Print and shaded views of the part. All mm, measured from the part's lowest x, y and z. Round coordinates to 2 decimals unless told otherwise and drop trailing zeros. Write each loop counter-clockwise with the first axis right and the second up, starting at its lowest first coordinate (ties: lowest second). Pieces come first, ordered by that corner, then holes. Notation, with made-up numbers: (-30, 56) -> (-6, 56) arc R17 cw to (-6, 79) -> close; hole circle Ø3 at (43, 85.25). An arc over 180 degrees is marked (long way). Return JSON: item names as keys, results as strings. Group by question number.
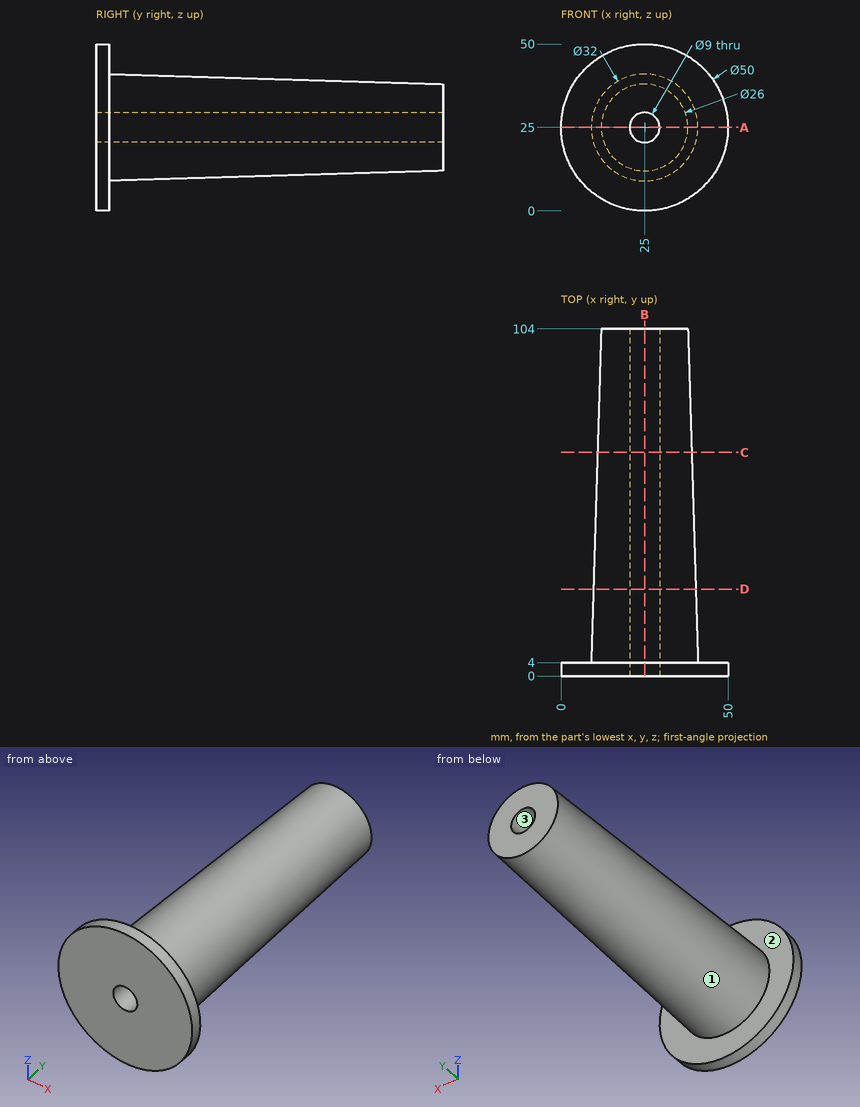
Item 1: Wall check: L1, parallel to Y at x = 39, z = 34; L2, parallel to Z at x = 25, y = 44; L3, parallel to X at y = 33, z = 25. Give the ranges that are in metal, low to high.
Item 2: Cut at C-C (y = 67). Write the cut outline in (x, z).
Item 3: Cut at A-A (z = 25). Write the cut outline in (x, y).
Item 4: Two-plate mould, pull along Z, no slides. Class the marked faces 1, 2 and 3: released by +Z, released by -Z, zero draft, split by the parting line, or undercut.
Item 5: Cut at D-D (y = 26). Write the cut outline in (x, z), then the cut area to 3 significant figures.
Item 6: Flat gauge pins, fed straight in: P1, Ø12, axis at y = 87.5, z = 23.5, coming from the -X side; P2, Ø2, axis at y = 90, z = 14, coming from the +X side; P3, Ø5, axis at y = 34, z = 29, coming from the -X side; P4, Ø7, axis at x = 25, z = 25, coming from the +Y side. Where does each tip first touch, or does it go through?
Item 7: Cut at B-B (x = 25). Write the cut outline in (y, z), then the cut area to 3 significant figures.
Checks:
{
 "1": {"L1": "y = 0 to 4", "L2": "z = 10.2 to 20.5, 29.5 to 39.8", "L3": "x = 9.87 to 20.5, 29.5 to 40.13"},
 "2": {"outline": "circle Ø28.22 at (25, 25); hole circle Ø9 at (25, 25)"},
 "3": {"outline": "(0, 0) -> (20.5, 0) -> (20.5, 104) -> (12, 104) -> (9, 4) -> (0, 4) -> close; (29.5, 0) -> (50, 0) -> (50, 4) -> (41, 4) -> (38, 104) -> (29.5, 104) -> close"},
 "4": {"face 1": "split by the parting line", "face 2": "zero draft", "face 3": "undercut"},
 "5": {"outline": "circle Ø30.68 at (25, 25); hole circle Ø9 at (25, 25)", "area": "676 mm2"},
 "6": {"P1": "stops at x = 11.33", "P2": "stops at x = 33.95", "P3": "stops at x = 9.96", "P4": "passes through"},
 "7": {"outline": "(0, 0) -> (4, 0) -> (4, 9) -> (104, 12) -> (104, 20.5) -> (0, 20.5) -> close; (0, 29.5) -> (104, 29.5) -> (104, 38) -> (4, 41) -> (4, 50) -> (0, 50) -> close", "area": "2,160 mm2"}
}
